Job drawing, mm, ordinate dimensions from the low corner. One solid piece. Give positions to 0.01 mm unless a question says otherwise; leave off trailing zeros. Loops run counter-clockwise (first coordinate to the right, second up) from the corner with the lowest first, then second, coordinate; pieces in that order, holes last. Notation, with made-up numbers: M 54.25,83 L 88.25,83 A28 ccw 88.25,116 Z; hole C 73.25,80 d2. An arc over 180 degrees is marked long. Answer in a Markdown table with one row per item.
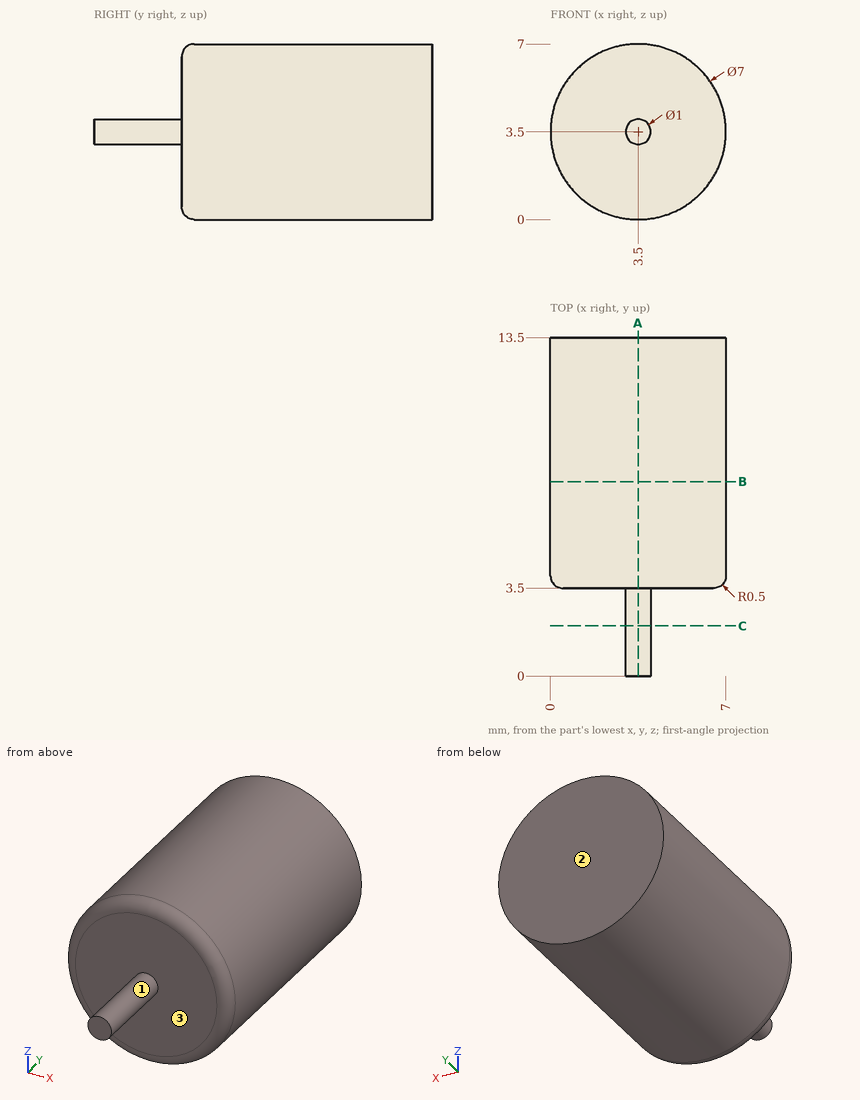
(1) Saw through at C-C (y = 2). Write the cut outline in (x, z), plus the area to 3 significant figures.
Recorded:
| item | result |
|---|---|
| outline | C 3.5,3.5 d1 |
| area | 0.785 mm^2 |
(2) Pull direction Y, two halves, no side cores. Call the marked faces 1, 2 and 3: +Y half, -Y half, draft (parallel to the pull), parting line (faces both ways), or undercut.
Recorded:
| item | result |
|---|---|
| face 1 | draft |
| face 2 | +Y half |
| face 3 | -Y half |
(3) Saw through at A-A (x = 3.5). Write the cut outline in (y, z).
Recorded:
| item | result |
|---|---|
| outline | M 0,3 L 3.5,3 L 3.5,0.5 A0.5 ccw 4,0 L 13.5,0 L 13.5,7 L 4,7 A0.5 ccw 3.5,6.5 L 3.5,4 L 0,4 Z |
(4) Saw through at B-B (y = 7.75). Write the cut outline in (x, z).
Recorded:
| item | result |
|---|---|
| outline | C 3.5,3.5 d7 |
(5) Drill centre lines: line 1 along Y through (x, z) = (2.5, 5.75); line 2 along X through (y, z) = (7.5, 5.25); line 3 along X through (y, z) = (4, 2.75). Where is each one in solid material? Low to high.
Recorded:
| item | result |
|---|---|
| line 1 | y = 3.5 to 13.5 |
| line 2 | x = 0.47 to 6.53 |
| line 3 | x = 0.08 to 6.92 |
(6) Pin check, flat tips, straight feed: pin 1 Ø1 at (y, z) = (7, 2) entering from +X; pin 2 Ø2 at (x, y) = (2, 3) entering from -Z. Stop position of each tip, or through.
Recorded:
| item | result |
|---|---|
| pin 1 | stops at x = 6.85 |
| pin 2 | stops at z = 0.16 |
